Here's how the part is built. I have some questions about the finished solid (model axes, mm). Face numbers are marked on the shaded views. Coordinates: 2 decimals unless noted, no trailing zeros. Loops run counter-clockwise (first coordinate to the right, second up) from the corner with the lowest first, then second, coordinate; pieces in that order, holes last. Notation, with made-up numbers: M 9,11.25 L 17,11.25 A20 ccw 17,31.25 Z; hole C 18,2 d5. An arc over 180 degrees is marked long. Use CSV: the item, a comma, the result in double quotes. Start each with the question number.
Q1. If we section it at A-A (z = 0): Please give me the cut outline in (x, y), and give its area (3 significant figures).
Q2. For pin 1 Ø3 at (x, z) = (-4, 16.5) entering from +Y; pin 2 Ø1 at (y, z) = (-88, -0.5) entering from +X; pin 3 Ø4 at (y, z) = (-163, 1) entering from +X, each with a flat end and sliding along its axis, tell me the tip position at first contact or that it passes through.
Q3. If we mould it in two halves opening along Z, with no side actions, what happens to the marked faces 1, 2, 3 and 4? For each: +Z half, -Z half, draft (parallel to the pull), parting line (faces both ways), or undercut.
Q4. If we section it at B-B (y = -124.5): Please give me the cut outline in (x, z), and give its area (3 significant figures).
Q5. Please list where these lines run through material, in increasing order: probe 1 along Y at (x, z) = (-6.75, 3); probe 2 along Z at (x, y) = (-4.75, -80.5) (3 decimals); probe 3 along Z at (x, y) = (-5, -157.5). Write a range as [from, to].
Q6. If we section it at C-C (z = 16.5): Please give me the cut outline in (x, y), and give its area (3 significant figures).
from build123d import *

# Parameters (mm, degrees)
SKETCH_1_W          = 40
SKETCH_1_H          = 270
EXTRUDE_1_DEPTH     = 17
CUT_EXTRUDE_1_DEPTH = 6
SKETCH_3_W          = 152.274191223
SKETCH_3_H          = 354.870754653
CUT_EXTRUDE_2_DEPTH = 272.272925298
SKETCH_5_W          = 16
SKETCH_5_H          = 25
CUT_EXTRUDE_3_DEPTH = 40
SKETCH_6_R          = 5.25
CUT_EXTRUDE_4_DEPTH = 120
CUT_EXTRUDE_5_DEPTH = 6.05


with BuildPart() as part:
    # 스케치1 → 보스-돌출1 (new, symmetric)
    with BuildSketch(Plane(origin=(0, 0, 0), x_dir=(0, 0, -1), z_dir=(1, 0, 0))):
        with Locations((0, -135)):
            Rectangle(SKETCH_1_W, SKETCH_1_H)
    extrude(amount=EXTRUDE_1_DEPTH, both=True)

    # 스케치2 → 컷-돌출1 (cut, symmetric)
    with BuildSketch(Plane(origin=(0, 0, 0), x_dir=(0, 0, -1), z_dir=(1, 0, 0))):
        Polygon((-12.025, 0), (-12.025, -90.319763504), (-6, -150.319763504), (6, -150.319763504), (12.025, -90.319763504), (12.025, 0), align=None)
    extrude(amount=CUT_EXTRUDE_1_DEPTH, both=True, mode=Mode.SUBTRACT)

    # 스케치3 → 컷-돌출2 (cut, through all)
    with BuildSketch(Plane(origin=(0, 0, 0), x_dir=(0, 0, -1), z_dir=(1, 0, 0))):
        with Locations((9.80305952, -151.338432535)):
            Rectangle(SKETCH_3_W, SKETCH_3_H)
    extrude(amount=CUT_EXTRUDE_2_DEPTH, mode=Mode.SUBTRACT)

    # 스케치5 → 컷-돌출3 (cut)
    with BuildSketch(Plane(origin=(0, -142, 0), x_dir=(1, 0, 0), z_dir=(0, 1, 0))):
        Rectangle(SKETCH_5_W, SKETCH_5_H)
    extrude(amount=-CUT_EXTRUDE_3_DEPTH, mode=Mode.SUBTRACT)

    # 스케치6 → 컷-돌출4 (cut)
    with BuildSketch(Plane(origin=(0, -142, 0), x_dir=(1, 0, 0), z_dir=(0, 1, 0))):
        Circle(SKETCH_6_R)
    extrude(amount=-CUT_EXTRUDE_4_DEPTH, mode=Mode.SUBTRACT)

    # 스케치7 → 컷-돌출5 (cut, symmetric)
    with BuildSketch(Plane(origin=(0, 0, 0), x_dir=(0, 0, -1), z_dir=(1, 0, 0))):
        Polygon((-6.155859274, -80), (-36.714111957, -80), (-36.714111957, 2.042704012), (-12.025, 2.042704012), (-12.025, -59.533635609), (-6.155859274, -68.262005046), align=None)
        with BuildLine():
            Line((6.890709855, 1.954718535), (7.897215171, 1.181933858))
            ThreePointArc((7.897215171, 1.181933858), (9.176015746, -2.135086772), (12.576405499, -3.172056537))
            Line((12.576405499, -3.172056537), (24.789660635, -11.787916198))
            Line((24.789660635, -11.787916198), (24.789660635, 1.954718535))
            Line((24.789660635, 1.954718535), (6.890709855, 1.954718535))
        make_face()
    extrude(amount=CUT_EXTRUDE_5_DEPTH, both=True, mode=Mode.SUBTRACT)


solid = part.part
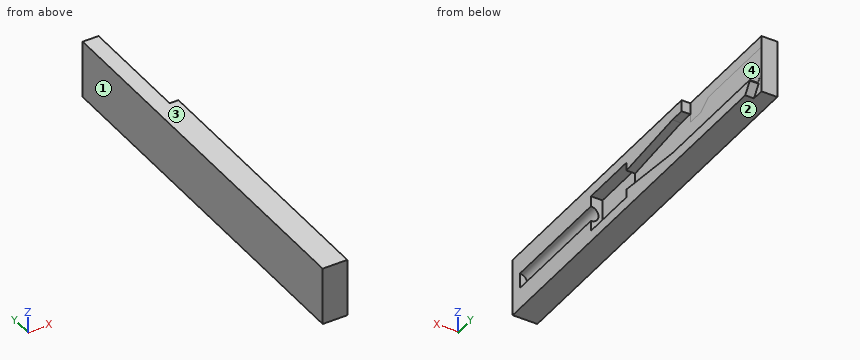
Results below:
1,outline,"M -17,-270 L 0,-270 L 0,-262 L -5.25,-262 L -5.25,-182 L -8,-182 L -8,-142 L -6,-142 L -6,0 L -17,0 Z"
1,area,"3,000 mm^2"
2,pin 1,"y = -80"
2,pin 2,"x = -6"
2,pin 3,"x = -8"
3,face 1,"draft"
3,face 2,"-Z half"
3,face 3,"+Z half"
3,face 4,"undercut"
4,outline,"M -17,-20 L 0,-20 L 0,-8.59 L -6,-8.59 L -6,8.59 L 0,8.59 L 0,20 L -17,20 Z"
4,area,"577 mm^2"
5,probe 1,"[-270, -182], [-142, 0]"
5,probe 2,"[-20, -12.025], [12.025, 20]"
5,probe 3,"[-20, -12.5], [12.5, 20]"
6,outline,"M -17,-270 L 0,-270 L 0,-80 L -6.05,-80 L -6.05,0 L -17,0 Z"
6,area,"4,110 mm^2"
